from build123d import *

# Parameters (mm, degrees)
SKETCH1_W           = 400
SKETCH1_H           = 300
SKETCH1_W_2         = 380
SKETCH1_H_2         = 280
BOSS_EXTRUDE1_DEPTH = 40
SKETCH4_R           = 3
BOSS_EXTRUDE4_DEPTH = 10
SKETCH2_R           = 3
CUT_EXTRUDE1_DEPTH  = 400


with BuildPart() as part:
    # Sketch1 → Boss-Extrude1 (new body)
    with BuildSketch(Plane(origin=(0, 0, 0), x_dir=(1, 0, 0), z_dir=(0, 1, 0))):
        Rectangle(SKETCH1_W, SKETCH1_H)
        Rectangle(SKETCH1_W_2, SKETCH1_H_2, mode=Mode.SUBTRACT)
    extrude(amount=BOSS_EXTRUDE1_DEPTH)

    # Sketch4 → Boss-Extrude4 (add)
    with BuildSketch(Plane.ZY.offset(200)):
        with Locations((110, 20)):
            Circle(SKETCH4_R)
    extrude(amount=BOSS_EXTRUDE4_DEPTH)

    # Sketch2 → Cut-Extrude1 (cut)
    with BuildSketch(Plane(origin=(200, 0, 0), x_dir=(0, 0, -1), z_dir=(1, 0, 0))):
        with Locations((0, 20)):
            Circle(SKETCH2_R)
    extrude(amount=-CUT_EXTRUDE1_DEPTH, mode=Mode.SUBTRACT)


solid = part.part
The listing builds one solid part. Answer for the finished solid, in the listing's coordinates (mm). A direction names the side the tool comes from. Round coordinates to 2 decimals unless told otherwise and drop trailing zeros. Order: outer loops, then holes, each group sorted by start corner. A loop starts at its lowest first (then second) coordinate and runs counter-clockwise, first axis right, second up. Notation, with made-up numbers: (-4, 84.25) - (31, 84.25) arc R16 ccw to (31, 109.25) - close; hole circle Ø1 at (-9, 64). An arc over 180 degrees is marked (long way). Write item = value, one per line. Start each with the question number.
1) For a pull along X with two mould halves and no side action, classify faces 3 (the flat face through (-200, 24, 2)), 4 (the flat face through (200, 24, 2)), 5 (the flat face through (-3, 20, -140)) as released by +X, released by -X, zero draft, split by the parting line, or undercut.
2) Section A-A, the plane x = 172 is taken. Write down the section's boundary in (y, z).
3) Given pin 1 (12 mm diameter, centred on y = 9.5, z = -69, fed in from -X); pin 2 (5.5 mm diameter, centred on y = 20, z = 0, fed in from +X); pin 3 (7 mm diameter, centred on y = 20, z = 0, fed in from +X), each flat-ended and moving along its own axis, determine where each tip first touches the part or whether it passes through.
4) Section C-C, the plane z = 124 is taken. Write down the section's boundary in (x, y), plus the area to 3 significant figures.
5) Straight lines are drawn through the part: L1, parallel to X at y = 21, z = -37; L2, parallel to Z at x = -55, y = 8; L3, parallel to Y at x = 197, z = 0. For each, find the intervals that lie inside material, in ascending order.
6) Section B-B, the plane y = 11 is taken. Write down the section's boundary in (x, z), plus the area to 3 significant figures.
7) For faces 1 (the flat face through (-190, 24, 2)), 2 (the flat face through (-3, 20, 150)), determine the directions among +Z, -Z, +X, -X, +Y, -Y from which every point of the face is accessible in a straight line to the end or side of a thin tool.
Results list:
q1.face_3 = released by -X
q1.face_4 = released by +X
q1.face_5 = undercut
q2.outline = (0, -150) - (40, -150) - (40, -140) - (0, -140) - close; (0, 140) - (40, 140) - (40, 150) - (0, 150) - close
q3.pin_1 = -200
q3.pin_2 = through
q3.pin_3 = 200
q4.outline = (-200, 0) - (-190, 0) - (-190, 40) - (-200, 40) - close; (190, 0) - (200, 0) - (200, 40) - (190, 40) - close
q4.area = 800 mm^2
q5.L1 = -200 to -190, 190 to 200
q5.L2 = -150 to -140, 140 to 150
q5.L3 = 0 to 17, 23 to 40
q6.outline = (-200, -150) - (200, -150) - (200, 150) - (-200, 150) - close; hole (-190, -140) - (190, -140) - (190, 140) - (-190, 140) - close
q6.area = 13,600 mm^2
q7.face_1 = +Y, -Y
q7.face_2 = +Z, +X, -X, +Y, -Y
